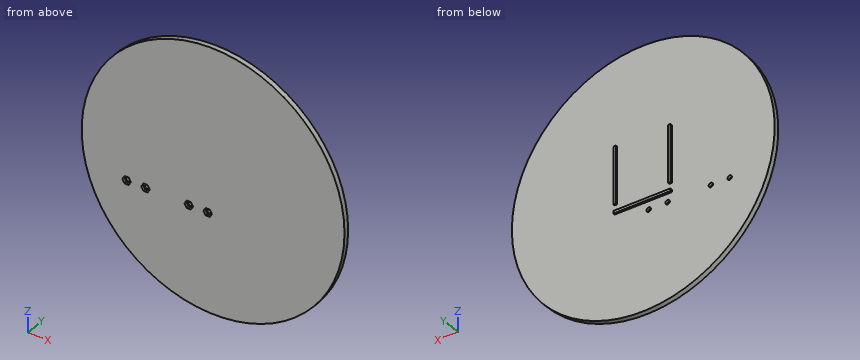
from build123d import *

# Parameters (mm, degrees)
SKETCH2_R           = 101.5
BOSS_EXTRUDE2_DEPTH = 2
SKETCH4_W           = 44.25
SKETCH4_H           = 2
SKETCH4_W_2         = 2
SKETCH4_H_2         = 44.25
BOSS_EXTRUDE3_DEPTH = 1.5
SKETCH5_R           = 1.7
CUT_EXTRUDE1_DEPTH  = 5
CUT_EXTRUDE2_DEPTH  = 2


with BuildPart() as part:
    # Sketch2 → Boss-Extrude2 (new body, symmetric)
    with BuildSketch(Plane(origin=(0, 0, 0), x_dir=(1, 0, 0), z_dir=(0, 1, 0))):
        Circle(SKETCH2_R)
    extrude(amount=BOSS_EXTRUDE2_DEPTH, both=True)

    # Sketch4 → Boss-Extrude3 (add, symmetric)
    with BuildSketch(Plane(origin=(0, 2, 0), x_dir=(1, 0, 0), z_dir=(0, 1, 0))):
        with Locations((0, 18)):
            Rectangle(SKETCH4_W, SKETCH4_H)
        with Locations((-21.125, -10.125)):
            Rectangle(SKETCH4_W_2, SKETCH4_H_2)
        with Locations((21.125, -10.125)):
            Rectangle(SKETCH4_W_2, SKETCH4_H_2)
    extrude(amount=BOSS_EXTRUDE3_DEPTH, both=True)

    # Sketch5 → Cut-Extrude1 (cut, through all)
    with BuildSketch(Plane(origin=(0, 2, 0), x_dir=(1, 0, 0), z_dir=(0, 1, 0))):
        with Locations((-66.8, 25.4)):
            Circle(SKETCH5_R)
        with Locations((-52.2, 25.4)):
            Circle(SKETCH5_R)
        with Locations((-18.8, 25.4)):
            Circle(SKETCH5_R)
        with Locations((-4.2, 25.4)):
            Circle(SKETCH5_R)
    extrude(amount=-CUT_EXTRUDE1_DEPTH, mode=Mode.SUBTRACT)

    # Sketch6 → Cut-Extrude2 (cut)
    with BuildSketch(Plane(origin=(0, -2, 0), x_dir=(-1, 0, 0), z_dir=(0, -1, 0))):
        Polygon((7.490896534, 25.4), (5.845448267, 28.25), (2.554551733, 28.25), (0.909103466, 25.4), (2.554551733, 22.55), (5.845448267, 22.55), align=None)
        Polygon((22.090896534, 25.4), (20.445448267, 28.25), (17.154551733, 28.25), (15.509103466, 25.4), (17.154551733, 22.55), (20.445448267, 22.55), align=None)
        Polygon((55.490896534, 25.4), (53.845448267, 28.25), (50.554551733, 28.25), (48.909103466, 25.4), (50.554551733, 22.55), (53.845448267, 22.55), align=None)
        Polygon((70.090896534, 25.4), (68.445448267, 28.25), (65.154551733, 28.25), (63.509103466, 25.4), (65.154551733, 22.55), (68.445448267, 22.55), align=None)
    extrude(amount=-CUT_EXTRUDE2_DEPTH, mode=Mode.SUBTRACT)


solid = part.part
Could you check a few things on this model? Use its own coordinates, in mm. Give positions to 0.01 mm unless a question says otherwise; leave off trailing zeros. Order: outer loops, then holes, each group sorted by start corner. A loop starts at its lowest first (then second) coordinate and runs counter-clockwise, first axis right, second up. Notation, with made-up numbers: (-26, 54) - (17, 54) arc R23 cw to (17, 87) - close; hole circle Ø8 at (76.25, 30.25). An arc over 180 degrees is marked (long way). One line per item, written item: value. Start each with the question number.
1. If I drill on probe 1 along X at (y, z) = (1.4, -25.4); probe 2 along Z at (x, y) = (20.5, 2.25); probe 3 along Y at (x, z) = (-18.5, 84.5), over which ranges is the centre line in solid material (lowest first)?
2. Imagine slicing it at C-C on x = 87. List the corners of the cut face in (y, z) for me.
3. Imagine slicing it at B-B on z = 12.5. List the corners of the cut face in (x, y) for me (3 decimals).
4. Imagine slicing it at A-A on y = -0.95. List the corners of the cut face in (x, z) for me, plus the area to 3 significant figures.
5. Imagine slicing it at D-D on x = -76. List the corners of the cut face in (y, z) for me, plus the area to 3 significant figures.
6. For P1, Ø2, axis at x = -66, y = -1, coming from the -Z side; P2, Ø6, axis at x = 13.5, z = -46.5, coming from the +Y side; P3, Ø1.6, axis at x = -52, y = -1, coming from the -Z side, each with a flat end and sliding along its axis, tell me the tip position at first contact or that it passes through.
Values:
1. probe 1: -98.27 to -68.5, -65.1 to -53.9, -50.5 to -20.5, -17.1 to -5.9, -2.5 to 98.27
1. probe 2: -19 to -17, -12 to 32.25
1. probe 3: -2 to 2
2. outline: (-2, -52.28) - (2, -52.28) - (2, 52.28) - (-2, 52.28) - close
3. outline: (-100.727, -2) - (100.727, -2) - (100.727, 2) - (22.125, 2) - (22.125, 3.5) - (20.125, 3.5) - (20.125, 2) - (-20.125, 2) - (-20.125, 3.5) - (-22.125, 3.5) - (-22.125, 2) - (-100.727, 2) - close
4. outline: circle Ø203 at (0, 0); hole (-70.09, -25.4) - (-68.45, -28.25) - (-65.15, -28.25) - (-63.51, -25.4) - (-65.15, -22.55) - (-68.45, -22.55) - close; hole (-55.49, -25.4) - (-53.85, -28.25) - (-50.55, -28.25) - (-48.91, -25.4) - (-50.55, -22.55) - (-53.85, -22.55) - close; hole (-22.09, -25.4) - (-20.45, -28.25) - (-17.15, -28.25) - (-15.51, -25.4) - (-17.15, -22.55) - (-20.45, -22.55) - close; hole (-7.49, -25.4) - (-5.85, -28.25) - (-2.55, -28.25) - (-0.91, -25.4) - (-2.55, -22.55) - (-5.85, -22.55) - close
4. area: 32,300 mm²
5. outline: (-2, -67.28) - (2, -67.28) - (2, 67.28) - (-2, 67.28) - close
5. area: 538 mm²
6. P1: z = -77.96
6. P2: y = 2
6. P3: z = -87.64
